Read the model definition and answer for the solid it produces. Units are mm, in the model's axes. Round coordinates to 2 decimals unless told otherwise and drop trailing zeros. Order: outer loops, then holes, each group sorted by start corner. A loop starts at its lowest first (then second) coordinate and runs counter-clockwise, first axis right, second up. Notation, with made-up numbers: (-2.75, 72.5) -> (53.25, 72.5) arc R24 cw to (53.25, 109.5) -> close; hole circle Ø7 at (9.5, 75). An arc over 180 degrees is marked (long way). Answer as a JSON object with one key per item and string values. Group by question number.
Item 1: Given P1, Ø1, axis at x = 15, z = -1, coming from the -Y side, flat-ended and moving along its own axis, determine where the tip first touches the part or whether it passes through.
Item 2: Consider probe 1 along X at (y, z) = (44, 0.6); probe 2 along X at (y, z) = (37, -0.45). Determine where each line is inside the solid, lowest interval first. Write a range as from..to.
Item 3: Section B-B, the plane y = 47.5 is taken. Write down the section's boundary in (x, z).
Item 4: Section A-A, the plane z = 0.15 is taken. Write down the section's boundary in (x, y).
from build123d import *

# Parameters (mm, degrees)
BOSS_EXTRUDE1_DEPTH = 52.5
CUT_EXTRUDE1_DEPTH  = 63.327762674


with BuildPart() as part:
    # Sketch2 → Boss-Extrude1 (new body)
    with BuildSketch(Plane(origin=(0, 0, 0), x_dir=(1, 0, 0), z_dir=(0, 1, 0))):
        Polygon((-31, 1.25), (-33.5, -1.25), (33.5, -1.25), (31, 1.25), align=None)
    extrude(amount=BOSS_EXTRUDE1_DEPTH)

    # Sketch3 → Cut-Extrude1 (cut, through all)
    with BuildSketch(Plane.XY.offset(1.25)):
        with BuildLine():
            ThreePointArc((0, 8.6), (-1.6, 7), (0, 5.4))
            Line((0, 5.4), (0, 8.6))
        make_face()
        with BuildLine():
            Line((0, 8.6), (0, 5.4))
            ThreePointArc((0, 5.4), (1.13137085, 5.86862915), (1.6, 7))
            ThreePointArc((1.6, 7), (1.13137085, 8.13137085), (0, 8.6))
        make_face()
    extrude(amount=-CUT_EXTRUDE1_DEPTH, mode=Mode.SUBTRACT)


solid = part.part
Values found:
{
 "1": {"P1": "y = 0"},
 "2": {"probe 1": "-32.85..32.85", "probe 2": "-31.8..31.8"},
 "3": {"outline": "(-33.5, 1.25) -> (-31, -1.25) -> (31, -1.25) -> (33.5, 1.25) -> close"},
 "4": {"outline": "(-32.4, 0) -> (32.4, 0) -> (32.4, 52.5) -> (-32.4, 52.5) -> close; hole circle Ø3.2 at (0, 7)"}
}
